from build123d import *

# Parameters (mm, degrees)
SKETCH_1_W      = 1
SKETCH_1_H      = 50
SKETCH_5_R      = 1.5
EXTRUDE_4_DEPTH = 50


with BuildPart() as part:
    # 草图1 → 旋转1 (revolve)
    with BuildSketch(Plane.XZ, mode=Mode.PRIVATE) as revolve_1_sk:
        with Locations((2, 25)):
            Rectangle(SKETCH_1_W, SKETCH_1_H)
    revolve(revolve_1_sk.sketch.rotate(Axis((0, 0, 50), (0, 0, -1)), 180), axis=Axis((0, 0, 50), (0, 0, -1)))

    # 草图5 → 凸台-拉伸4 (add)
    with BuildSketch(Plane(origin=(0, 0, 0), x_dir=(-1, 0, 0), z_dir=(0, 0, -1))):
        Polygon((-1.504244122, 2.59562124), (-2.999995993, -0.004903003), (-1.495751872, -2.600524243), (1.504244122, -2.59562124), (2.999995993, 0.004903003), (1.495751872, 2.600524243), align=None)
        Circle(SKETCH_5_R, mode=Mode.SUBTRACT)
    extrude(amount=-EXTRUDE_4_DEPTH)


solid = part.part
Design review of the part built by this model. Coordinates are the model's own, in mm. Coordinates: 2 decimals unless noted, no trailing zeros. Loops run counter-clockwise (first coordinate to the right, second up) from the corner with the lowest first, then second, coordinate; pieces in that order, holes last. Notation, with made-up numbers: M -9.5,-21 L 42.5,-21 A30 cw 42.5,1 Z; hole C 50.5,42.25 d10. An arc over 180 degrees is marked long. Answer as CSV lines item,"result".
Item 1: For P1, Ø1.5, axis at x = -1.5, z = 26, coming from the -Y side, flat-tipped, find the tip position at first contact; note if it passes through.
Answer list:
P1,"y = -2.6"
Item 2: Add section B-B on z = 32. State the section outline as (x, y) points.
Answer list:
outline,"M -3,0 L -1.5,-2.6 L 1.5,-2.6 L 3,0 L 1.5,2.6 L -1.5,2.6 Z; hole C 0,0 d3"
Item 3: For probe 1 along Y at (x, z) = (0, 16.5); probe 2 along Y at (x, z) = (-1.15, 39); probe 3 along X at (y, z) = (0.95, 39.5), list the stretches that pass through material, from the lowest coordinate up.
Answer list:
probe 1,"-2.6 to -1.5, 1.5 to 2.6"
probe 2,"-2.6 to -0.96, 0.96 to 2.6"
probe 3,"-2.45 to -1.16, 1.16 to 2.45"
Item 4: Add section D-D on x = 2.45. State the section outline as (y, z) points.
Answer list:
outline,"M -0.95,0 L 0.95,0 L 0.95,50 L -0.95,50 Z"
Item 5: The part is to be moulded in two halves that separate along Y. For faces 1 (the face through (-1.3, 1.2, 50)), 2 (the face through (-1.43, 0.45, 25.35)), 3 (the face through (-2.242, -1.314, 24.65)), say which applies: pulls with the +Y half, pulls with the -Y half, needs draft (parallel to the pull), parting line crosses it, or undercut.
Answer list:
face 1,"needs draft"
face 2,"undercut"
face 3,"pulls with the -Y half"
Item 6: Add section C-C on y = -0.6. State the section outline as (x, z) points, plus the area to 3 significant figures.
Answer list:
outline,"M -2.65,0 L -1.37,0 L -1.37,50 L -2.65,50 Z; M 1.37,0 L 2.66,0 L 2.66,50 L 1.37,50 Z"
area,"128 mm²"
Item 7: Add section A-A on x = 0. State the section outline as (y, z) points.
Answer list:
outline,"M -2.6,0 L -1.5,0 L -1.5,50 L -2.6,50 Z; M 1.5,0 L 2.6,0 L 2.6,50 L 1.5,50 Z"
